Geometry check sheet. Reference: the model listing, model coordinates, mm. Give positions to 0.01 mm unless a question says otherwise; leave off trailing zeros. Loops run counter-clockwise (first coordinate to the right, second up) from the corner with the lowest first, then second, coordinate; pieces in that order, holes last. Notation, with made-up numbers: (78, 62.25) -> (130, 62.25) arc R24 cw to (130, 101.25) -> close; hole circle Ø4 at (-6, 82). An arc over 180 degrees is marked (long way). Answer as a JSON object with one key per item and string values.
from build123d import *

# Parameters (mm, degrees)
F0_R     = 2.247709
F1_DEPTH = 1.27
F2_R     = 5.08


with BuildPart() as f1:
    # F0 (on Front) → F1 (new body)
    with BuildSketch(Plane.XZ):
        Polygon((0, -50.8), (0, 0), (0, 50.8), (-50.8, 50.8), (-50.8, 0), (-50.8, -50.8), align=None)
        with Locations((-25.4, 44.52955)):
            Circle(F0_R, mode=Mode.SUBTRACT)
    extrude(amount=F1_DEPTH)

    # F2
    f2_edges = [f1.edges().sort_by_distance(p)[0] for p in [
        (0, -0.635, 50.8),
        (-50.8, -0.635, 50.8),
        (-50.8, -0.635, -50.8),
        (0, -0.635, -50.8),
    ]]
    fillet(f2_edges, radius=F2_R)


solid = f1.part
1) Material ranges on line 1 along Z through (x, y) = (-25.4, -0.95); line 2 along Z through (x, y) = (-25, -0.75); line 3 along X through (y, z) = (-0.8, 46.5), recorded low to high. Write a range as from..to.
Geometry check:
{"line 1": "z = -50.8..42.28, 46.78..50.8", "line 2": "z = -50.8..42.32, 46.74..50.8", "line 3": "x = -50.74..-26.48, -24.32..-0.06"}
2) Depth check by flat-ended pin: P1, Ø2.5, axis at x = -25.4, z = 44.53, coming from the -Y side. Enter the tip coordinate at first touch or a pass-through.
Geometry check:
{"P1": "passes through"}
3) Draft check along Z on faces 1 (the face through (-27.18, -0.63, 43.16)), 2 (the face through (-49.272, -0.644, 49.351)), 3 (the face through (-26, 0, 1)). Enter one of: pulls with the +Z half, pulls with the -Z half, needs draft (parallel to the pull), parting line crosses it, or undercut.
Geometry check:
{"face 1": "undercut", "face 2": "pulls with the +Z half", "face 3": "needs draft"}
4) Section check A-A on x = -25.4. Record the cut outline in (y, z), plus the area to 3 significant figures.
Geometry check:
{"outline": "(-1.27, -50.8) -> (0, -50.8) -> (0, 42.28) -> (-1.27, 42.28) -> close; (-1.27, 46.78) -> (0, 46.78) -> (0, 50.8) -> (-1.27, 50.8) -> close", "area": "123 mm2"}
